from build123d import *

# Parameters (mm, degrees)
SKETCH_W     = 50
SKETCH_H     = 48
SKETCH_R     = 1.4
PAD_DEPTH    = 2
SKETCH003_R  = 1.4
PAD001_DEPTH = 2
SKETCH004_R  = 3.5
PAD002_DEPTH = 2
FILLET_R     = 1
FILLET001_R  = 1


with BuildPart() as part:
    # Sketch → Pad (new body)
    with BuildSketch(Plane.XZ):
        Rectangle(SKETCH_W, SKETCH_H)
        with Locations((-5, 5)):
            Circle(SKETCH_R, mode=Mode.SUBTRACT)
        with Locations((5, 5)):
            Circle(SKETCH_R, mode=Mode.SUBTRACT)
        with Locations((-5, -5)):
            Circle(SKETCH_R, mode=Mode.SUBTRACT)
        with Locations((5, -5)):
            Circle(SKETCH_R, mode=Mode.SUBTRACT)
        Circle(SKETCH_R, mode=Mode.SUBTRACT)
    extrude(amount=PAD_DEPTH)

    # Sketch003 (on Face3 of Pad) → Pad001 (join)
    with BuildSketch(Plane(origin=(0, 0, -24), x_dir=(1, 0, 0), z_dir=(0, 0, -1))):
        with BuildLine():
            Line((-25, 0), (-25, 2))
            Line((-25, 2), (25, 2))
            Line((25, 2), (25, 0))
            Line((25, 0), (25, -5))
            Line((25, -5), (20.80638, -27.054785))
            ThreePointArc((1.756653, -32.283353), (12.911489, -35.607697), (20.80638, -27.054785))
            Line((-25, -2), (1.756653, -32.283353))
            Line((-25, 0), (-25, -2))
        make_face()
        with Locations((10, -31.934549)):
            Circle(SKETCH003_R, mode=Mode.SUBTRACT)
        with Locations((17.205, -25)):
            Circle(SKETCH003_R, mode=Mode.SUBTRACT)
        with Locations((10, -25)):
            Circle(SKETCH003_R, mode=Mode.SUBTRACT)
        with Locations((2.795, -25)):
            Circle(SKETCH003_R, mode=Mode.SUBTRACT)
        with Locations((10, -18.065451)):
            Circle(SKETCH003_R, mode=Mode.SUBTRACT)
    extrude(amount=PAD001_DEPTH)

    # Sketch004 (on Face1 of Pad) → Pad002 (join)
    with BuildSketch(Plane(origin=(0, 0, 24), x_dir=(-1, 0, 0), z_dir=(0, 0, 1))):
        with BuildLine():
            Line((-25, 2), (25, 2))
            Line((25, 2), (25, 0))
            Line((25, 0), (25, -2))
            Line((25, -2), (-1.756653, -32.283353))
            ThreePointArc((-20.80638, -27.054785), (-12.911489, -35.607697), (-1.756653, -32.283353))
            Line((-25, -5), (-20.80638, -27.054785))
            Line((-25, 0), (-25, -5))
            Line((-25, 0), (-25, 2))
        make_face()
        with Locations((-10, -25)):
            Circle(SKETCH004_R, mode=Mode.SUBTRACT)
    extrude(amount=PAD002_DEPTH)

    # Fillet
    fillet_edges = [part.edges().sort_by_distance(p)[0] for p in [
        (0, 0, 24),
    ]]
    fillet(fillet_edges, radius=FILLET_R)

    # Fillet001
    fillet001_edges = [part.edges().sort_by_distance(p)[0] for p in [
        (0, 0, -24),
    ]]
    fillet(fillet001_edges, radius=FILLET001_R)


solid = part.part
The model under review builds one solid part; all positions refer to its coordinate system, in mm. A direction names the side the tool comes from. Round coordinates to 2 decimals unless told otherwise and drop trailing zeros. Order: outer loops, then holes, each group sorted by start corner. A loop starts at its lowest first (then second) coordinate and runs counter-clockwise, first axis right, second up. Notation, with made-up numbers: (44.25, 26) -> (98.25, 26) arc R21 ccw to (98.25, 60) -> close; hole circle Ø11 at (40, -36.75). An arc over 180 degrees is marked (long way). Write item = value, one per line. Start each with the question number.
Item 1: Mouldability with a two-part tool opening along Y and no side actions: class faces 4 (the face through (22.933, 15.873, 24.986)), 5 (the face through (10.46, 21.53, 24.99)), 6 (the face through (-25, -1, 0)) as released by +Y, released by -Y, zero draft, split by the parting line, or undercut.
Item 2: Consider section C-C on x = -5. Write out the cut boundary in (y, z).
Item 3: For line 1 along Z through (x, y) = (-5, -1.4); line 2 along Z through (x, y) = (2.5, 19); line 3 along X through (y, z) = (25, -24.9) (1 decimal), list the stretches that pass through material, from the lowest coordinate up.
Item 4: Consider section A-A on x = 10. Write out the cut boundary in (y, z).
Item 5: Consider section D-D on y = 25. Write out the cut boundary in (x, z) (1 decimal), plus the area to 3 significant figures.
Item 6: For faces 1 (the face through (-3.71, -0.99, -5.54)), 2 (the face through (5, 14, 24)), 3 (the face through (9.818, 30.546, -24.986)), list the 3-axis set-ups (+Z, -Z, +X, -X, +Y, -Y) from which the entire face can be reached by the end or side of a thin tool; tool diameter is ignored.
Item 7: Consider section B-B on z = 0. Write out the cut boundary in (x, y).
Item 8: Clearance check with flat-ended pins moving along their axes: pin 1 Ø2.5 at (x, z) = (5, 5) entering from -Y; pin 2 Ø3 at (x, z) = (5, -5) entering from -Y; pin 3 Ø3 at (x, z) = (-5, 5) entering from +Y; pin 4 Ø2.5 at (x, y) = (2.795, 25) entering from -Z. State where each tip first meets the part, or that it passes through.
Conclusion:
q1.face_4 = released by +Y
q1.face_5 = undercut
q1.face_6 = zero draft
q2.outline = (-2, -26) -> (24.64, -26) -> (24.64, -24) -> (1, -24) arc R1 cw to (0, -23) -> (0, -6.4) -> (-2, -6.4) -> close; (-2, -3.6) -> (0, -3.6) -> (0, 3.6) -> (-2, 3.6) -> close; (-2, 6.4) -> (0, 6.4) -> (0, 23) arc R1 cw to (1, 24) -> (24.64, 24) -> (24.64, 26) -> (-2, 26) -> close
q3.line_1 = -26 to -6.4, -3.6 to 3.6, 6.4 to 26
q3.line_2 = -26 to -24, 24 to 26
q3.line_3 = -4.7 to 1.4, 4.2 to 8.6, 11.4 to 15.8, 18.6 to 21.2
q4.outline = (-2, -26) -> (16.67, -26) -> (16.67, -24) -> (1, -24) arc R1 cw to (0, -23) -> (0, 23) arc R1 cw to (1, 24) -> (21.5, 24) -> (21.5, 26) -> (-2, 26) -> close; (19.47, -26) -> (23.6, -26) -> (23.6, -24) -> (19.47, -24) -> close; (26.4, -26) -> (30.53, -26) -> (30.53, -24) -> (26.4, -24) -> close; (28.5, 24) -> (36, 24) -> (36, 26) -> (28.5, 26) -> close; (33.33, -26) -> (36, -26) -> (36, -24) -> (33.33, -24) -> close
q5.outline = (-4.7, -26) -> (1.4, -26) -> (1.4, -24) -> (-4.7, -24) -> close; (-4.7, 24) -> (6.5, 24) -> (6.5, 26) -> (-4.7, 26) -> close; (4.2, -26) -> (8.6, -26) -> (8.6, -24) -> (4.2, -24) -> close; (11.4, -26) -> (15.8, -26) -> (15.8, -24) -> (11.4, -24) -> close; (13.5, 24) -> (21.2, 24) -> (21.2, 26) -> (13.5, 26) -> close; (18.6, -26) -> (21.2, -26) -> (21.2, -24) -> (18.6, -24) -> close
q5.area = 72.7 mm2
q6.face_1 = +Y, -Y
q6.face_2 = +X, -X, +Y
q6.face_3 = -Z
q7.outline = (-25, -2) -> (-1.4, -2) -> (-1.4, 0) -> (-25, 0) -> close; (1.4, -2) -> (25, -2) -> (25, 0) -> (1.4, 0) -> close
q8.pin_1 = through
q8.pin_2 = -2
q8.pin_3 = 0
q8.pin_4 = 24
